Autodesk Inventor part; units mm, degrees
ref_plane "YZ Plane" through (0, 0, 0) normal (1, 0, 0) x (0, 1, 0)
ref_plane "XZ Plane" through (0, 0, 0) normal (0, 1, 0) x (-1, 0, 0)
ref_plane "XY Plane" through (0, 0, 0) normal (0, 0, 1) x (1, 0, 0)
sketch "Sketch1" plane through (0, 0, 0) normal (0, 0, 1) x (1, 0, 0)
  line L0 (-102.5, -25) -> (102.5, -25)
  line L1 (102.5, -25) -> (102.5, 25)
  line L2 (102.5, 25) -> (-102.5, 25)
  line L3 (-102.5, 25) -> (-102.5, -25)
  line L4 (-102.5, -25) -> (102.5, 25) construction
  line L5 (102.5, -25) -> (-102.5, 25) construction
  point P0 (0, 0)
  dimension "d0" = 205
  dimension "d1" = 50
extrude "Plate1" add sketch "Sketch1" along normal blind 3
sketch "Sketch2" plane through (0, 0, 3) normal (0, 0, 1) x (1, 0, 0)
  line L0 (102.5, 25) -> (-102.5, 25)
  line L1 (47.5, 25) -> (52.5, 25)
  line L2 (52.5, 25) -> (52.5, 10)
  line L3 (52.5, 10) -> (47.5, 10)
  line L4 (47.5, 10) -> (47.5, 25)
  line L5 (102.5, 25) -> (102.5, -25)
  point P0 (0, 0)
  point P1 (52.5, 25)
  dimension "d3" = 50
  dimension "d4" = 5
  dimension "d5" = 15
extrude "Cut1" cut sketch "Sketch2" against normal blind 3
pattern_linear "Rectangular Pattern1" count 3 spacing 50 along (-1, 0, 0) of "Cut1"
equation "\"d6\" = Thickness"
equation "\"d2\" = Thickness"
equation "\"BendRadius\" = Thickness"
equation "\"BendReliefWidth\" = Thickness"
equation "\"BendReliefDepth\" = 0.5 * Thickness"
equation "\"CornerReliefSize\" = 4 * Thickness"
equation "\"MinimumRemnant\" = 2 * Thickness"
equation "\"TransitionRadius\" = BendRadius"
equation "\"JacobiRadiusSize\" = BendRadius"
equation "\"GapSize\" = Thickness"
properties part number "Sensors Shield"
The model under review builds one solid part; all positions refer to its coordinate system, in mm. Round coordinates to 2 decimals unless told otherwise and drop trailing zeros. Write each loop counter-clockwise with the first axis right and the second up, starting at its lowest first coordinate (ties: lowest second). Pieces come first, ordered by that corner, then holes. Notation, with made-up numbers: (43.5, 57.5) - (75.5, 57.5) arc R17 ccw to (75.5, 86.5) - close; hole circle Ø9 at (58.25, -3.75). An arc over 180 degrees is marked (long way). One line per item, written item: value. Start each with the question number.
1. To check wall thickness, follow L1, parallel to X at y = 20, z = 1.35; L2, parallel to Y at x = -48, z = 2.9. State the ranges of each line that lie inside material, in increasing order. Write a range as from..to.
2. Clearance check with a flat-ended pin moving along its axis: P1, Ø0.9, axis at x = 50.5, z = 2, coming from the +Y side. State where the tip first meets the part, or that it passes through.
3. Consider section A-A on y = 12.5. Write out the cut boundary in (x, z).
4. Consider section B-B on z = 1.4. Write out the cut boundary in (x, y), and give its area (3 significant figures).
Checks:
1. L1: x = -102.5..-52.5, -47.5..-2.5, 2.5..47.5, 52.5..102.5
1. L2: y = -25..10
2. P1: stops at y = 10
3. outline: (-102.5, 0) - (-52.5, 0) - (-52.5, 3) - (-102.5, 3) - close; (-47.5, 0) - (-2.5, 0) - (-2.5, 3) - (-47.5, 3) - close; (2.5, 0) - (47.5, 0) - (47.5, 3) - (2.5, 3) - close; (52.5, 0) - (102.5, 0) - (102.5, 3) - (52.5, 3) - close
4. outline: (-102.5, -25) - (102.5, -25) - (102.5, 25) - (52.5, 25) - (52.5, 10) - (47.5, 10) - (47.5, 25) - (2.5, 25) - (2.5, 10) - (-2.5, 10) - (-2.5, 25) - (-47.5, 25) - (-47.5, 10) - (-52.5, 10) - (-52.5, 25) - (-102.5, 25) - close
4. area: 10,000 mm^2
